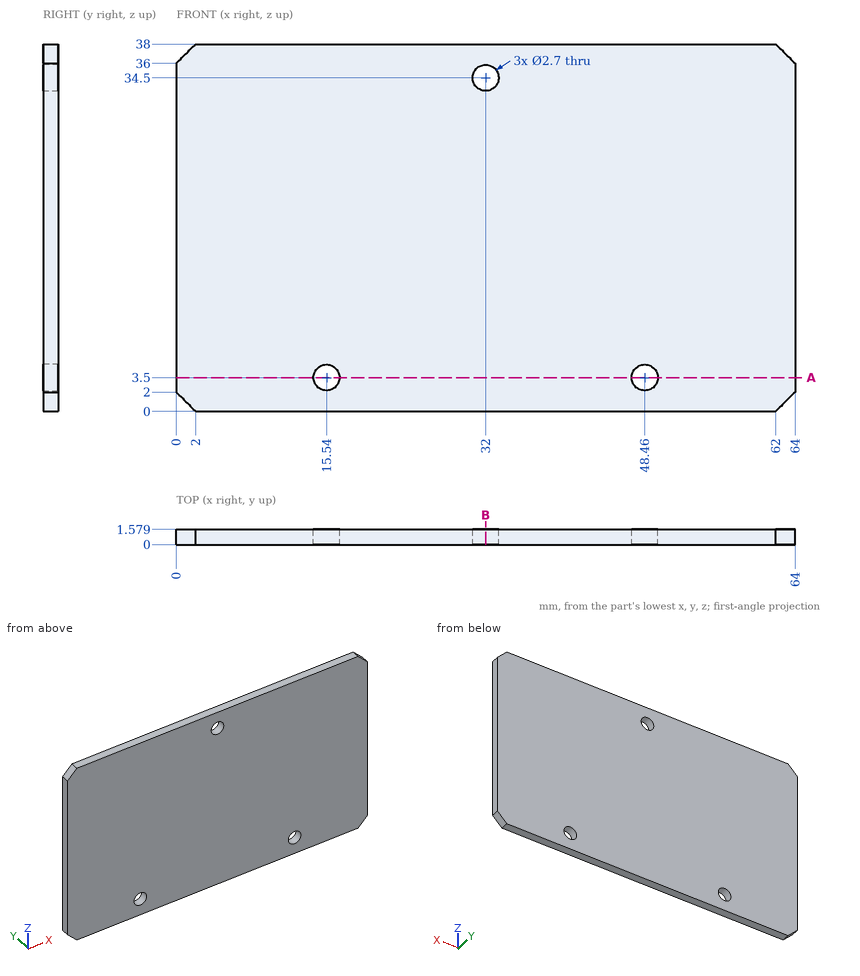
Check sheet for the drawn part. Datum: minimum x, y, z corner. Units: mm. Coordinates: 2 decimals unless noted, no trailing zeros. Order: outer loops, then holes, each group sorted by start corner. A loop starts at its lowest first (then second) coordinate and runs counter-clockwise, first axis right, second up. Notation, with made-up numbers: (-36.5, 16.5) - (-2.5, 16.5) arc R36 cw to (-2.5, 55.5) - close; hole circle Ø1 at (-38, 42.5). An arc over 180 degrees is marked (long way). Return JSON: item names as keys, results as strings.
(1) Section check B-B, the plane x = 32. Record the cut outline in (y, z).
Filled sheet:
{"outline": "(0, 0) - (1.58, 0) - (1.58, 33.15) - (0, 33.15) - close; (0, 35.85) - (1.58, 35.85) - (1.58, 38) - (0, 38) - close"}
(2) Section check A-A, the plane z = 3.5. Record the cut outline in (x, y).
Filled sheet:
{"outline": "(0, 0) - (14.19, 0) - (14.19, 1.58) - (0, 1.58) - close; (16.89, 0) - (47.11, 0) - (47.11, 1.58) - (16.89, 1.58) - close; (49.81, 0) - (64, 0) - (64, 1.58) - (49.81, 1.58) - close"}
(3) Thickness scan on line 1 along X through (y, z) = (0.9, 3.5); line 2 along Z through (x, y) = (15.54, 1.1); line 3 along X through (y, z) = (0.6, 34.5). Record the ranges inside material, lowest first.
Filled sheet:
{"line 1": "x = 0 to 14.19, 16.89 to 47.11, 49.81 to 64", "line 2": "z = 0 to 2.15, 4.85 to 38", "line 3": "x = 0 to 30.65, 33.35 to 64"}
